Here's how the part is built. I have some questions about the finished solid (model axes, mm). A direction names the side the tool comes from. Round coordinates to 2 decimals unless told otherwise and drop trailing zeros. Write each loop counter-clockwise with the first axis right and the second up, starting at its lowest first coordinate (ties: lowest second). Pieces come first, ordered by that corner, then holes. Notation, with made-up numbers: (-38.75, 11.5) -> (-14.75, 11.5) arc R26 cw to (-14.75, 34.5) -> close; hole circle Ø10 at (49, -37.5). An arc over 180 degrees is marked (long way). Answer in a Markdown table with one row per item. Add a question column.
from build123d import *

# Parameters (mm, degrees)
SKETCH2_W           = 130
SKETCH2_H           = 70
BOSS_EXTRUDE1_DEPTH = 100
SKETCH3_W           = 104
SKETCH3_H           = 74
CUT_EXTRUDE1_DEPTH  = 67
SKETCH4_W           = 10
SKETCH4_H           = 10
CUT_EXTRUDE2_DEPTH  = 55
SKETCH5_W           = 104
SKETCH5_H           = 10
CUT_EXTRUDE3_DEPTH  = 67
SKETCH6_W           = 10
SKETCH6_H           = 74
CUT_EXTRUDE4_DEPTH  = 67
SKETCH9_R           = 1.75
CUT_EXTRUDE5_DEPTH  = 67
SKETCH10_R          = 4
CUT_EXTRUDE6_DEPTH  = 5
SKETCH12_R          = 4
CUT_EXTRUDE7_DEPTH  = 5
SKETCH13_R          = 4
CUT_EXTRUDE8_DEPTH  = 5
SKETCH14_R          = 4
CUT_EXTRUDE9_DEPTH  = 5
SKETCH15_W          = 3
SKETCH15_H          = 3
BOSS_EXTRUDE2_DEPTH = 5
SKETCH16_W          = 76
SKETCH16_H          = 3
BOSS_EXTRUDE3_DEPTH = 15
SKETCH17_W          = 3
SKETCH17_H          = 30
BOSS_EXTRUDE4_DEPTH = 15
SKETCH18_R          = 5.8
CUT_EXTRUDE10_DEPTH = 15
SKETCH19_R          = 3.4
CUT_EXTRUDE11_DEPTH = 15


with BuildPart() as part:
    # Sketch2 → Boss-Extrude1 (new body)
    with BuildSketch(Plane(origin=(0, 0, 0), x_dir=(1, 0, 0), z_dir=(0, 1, 0))):
        with Locations((65, 35)):
            Rectangle(SKETCH2_W, SKETCH2_H)
    extrude(amount=BOSS_EXTRUDE1_DEPTH)

    # Sketch3 → Cut-Extrude1 (cut)
    with BuildSketch(Plane(origin=(0, 0, -70), x_dir=(-1, 0, 0), z_dir=(0, 0, -1))):
        with Locations((-65, 50)):
            Rectangle(SKETCH3_W, SKETCH3_H)
    extrude(amount=-CUT_EXTRUDE1_DEPTH, mode=Mode.SUBTRACT)

    # Sketch4 → Cut-Extrude2 (cut)
    with BuildSketch(Plane.XY):
        with Locations((5, 95)):
            Rectangle(SKETCH4_W, SKETCH4_H)
        with Locations((125, 95)):
            Rectangle(SKETCH4_W, SKETCH4_H)
        with Locations((5, 5)):
            Rectangle(SKETCH4_W, SKETCH4_H)
        with Locations((125, 5)):
            Rectangle(SKETCH4_W, SKETCH4_H)
    extrude(amount=-CUT_EXTRUDE2_DEPTH, mode=Mode.SUBTRACT)

    # Sketch5 → Cut-Extrude3 (cut)
    with BuildSketch(Plane(origin=(0, 0, -70), x_dir=(-1, 0, 0), z_dir=(0, 0, -1))):
        with Locations((-65, 92)):
            Rectangle(SKETCH5_W, SKETCH5_H)
        with Locations((-65, 8)):
            Rectangle(SKETCH5_W, SKETCH5_H)
    extrude(amount=-CUT_EXTRUDE3_DEPTH, mode=Mode.SUBTRACT)

    # Sketch6 → Cut-Extrude4 (cut)
    with BuildSketch(Plane(origin=(0, 0, -70), x_dir=(-1, 0, 0), z_dir=(0, 0, -1))):
        with Locations((-122, 50)):
            Rectangle(SKETCH6_W, SKETCH6_H)
        with Locations((-8, 50)):
            Rectangle(SKETCH6_W, SKETCH6_H)
    extrude(amount=-CUT_EXTRUDE4_DEPTH, mode=Mode.SUBTRACT)

    # Sketch9 → Cut-Extrude5 (cut)
    with BuildSketch(Plane(origin=(0, 0, -70), x_dir=(-1, 0, 0), z_dir=(0, 0, -1))):
        with Locations((-124, 94)):
            Circle(SKETCH9_R)
        with Locations((-124, 6)):
            Circle(SKETCH9_R)
        with Locations((-6, 94)):
            Circle(SKETCH9_R)
        with Locations((-6, 6)):
            Circle(SKETCH9_R)
    extrude(amount=-CUT_EXTRUDE5_DEPTH, mode=Mode.SUBTRACT)

    # Sketch10 → Cut-Extrude6 (cut)
    with BuildSketch(Plane.XY.offset(-55)):
        with Locations((124, 94)):
            Circle(SKETCH10_R)
    extrude(amount=-CUT_EXTRUDE6_DEPTH, mode=Mode.SUBTRACT)

    # Sketch12 → Cut-Extrude7 (cut)
    with BuildSketch(Plane.XY.offset(-55)):
        with Locations((124, 6)):
            Circle(SKETCH12_R)
    extrude(amount=-CUT_EXTRUDE7_DEPTH, mode=Mode.SUBTRACT)

    # Sketch13 → Cut-Extrude8 (cut)
    with BuildSketch(Plane.XY.offset(-55)):
        with Locations((6, 6)):
            Circle(SKETCH13_R)
    extrude(amount=-CUT_EXTRUDE8_DEPTH, mode=Mode.SUBTRACT)

    # Sketch14 → Cut-Extrude9 (cut)
    with BuildSketch(Plane.XY.offset(-55)):
        with Locations((6, 94)):
            Circle(SKETCH14_R)
    extrude(amount=-CUT_EXTRUDE9_DEPTH, mode=Mode.SUBTRACT)

    # Sketch15 → Boss-Extrude2 (add)
    with BuildSketch(Plane(origin=(0, 0, -70), x_dir=(-1, 0, 0), z_dir=(0, 0, -1))):
        with Locations((-118.5, 88.5)):
            Rectangle(SKETCH15_W, SKETCH15_H)
        with Locations((-118.5, 11.5)):
            Rectangle(SKETCH15_W, SKETCH15_H)
        with Locations((-11.5, 11.5)):
            Rectangle(SKETCH15_W, SKETCH15_H)
        with Locations((-11.5, 88.5)):
            Rectangle(SKETCH15_W, SKETCH15_H)
    extrude(amount=BOSS_EXTRUDE2_DEPTH)

    # Sketch16 → Boss-Extrude3 (add)
    with BuildSketch(Plane(origin=(0, 3, 0), x_dir=(1, 0, 0), z_dir=(0, 1, 0))):
        with Locations((79, 68.5)):
            Rectangle(SKETCH16_W, SKETCH16_H)
    extrude(amount=BOSS_EXTRUDE3_DEPTH)

    # Sketch17 → Boss-Extrude4 (add)
    with BuildSketch(Plane(origin=(0, 0, -3), x_dir=(-1, 0, 0), z_dir=(0, 0, -1))):
        with Locations((-99.5, 33)):
            Rectangle(SKETCH17_W, SKETCH17_H)
        with Locations((-36.5, 33)):
            Rectangle(SKETCH17_W, SKETCH17_H)
    extrude(amount=BOSS_EXTRUDE4_DEPTH)

    # Sketch18 → Cut-Extrude10 (cut)
    with BuildSketch(Plane(origin=(0, 0, -3), x_dir=(-1, 0, 0), z_dir=(0, 0, -1))):
        with Locations((-20, 25)):
            Circle(SKETCH18_R)
    extrude(amount=-CUT_EXTRUDE10_DEPTH, mode=Mode.SUBTRACT)

    # Sketch19 → Cut-Extrude11 (cut)
    with BuildSketch(Plane(origin=(0, 100, 0), x_dir=(1, 0, 0), z_dir=(0, 1, 0))):
        with Locations((25, 45)):
            Circle(SKETCH19_R)
        with Locations((45, 45)):
            Circle(SKETCH19_R)
        with Locations((65, 45)):
            Circle(SKETCH19_R)
        with Locations((85, 45)):
            Circle(SKETCH19_R)
        with Locations((105, 45)):
            Circle(SKETCH19_R)
    extrude(amount=-CUT_EXTRUDE11_DEPTH, mode=Mode.SUBTRACT)


solid = part.part
Item 1: I need wall thicknesses on line 1 along X through (y, z) = (99.3, -45); line 2 along X through (y, z) = (38, -17.5); line 3 along X through (y, z) = (54, -17). Which ranges of each line are inside material? Lowest first, please. Write a range as from..to.
Item 2: If we section it at C-C on x = 65: Please give me the cut outline in (y, z).
Item 3: If we section it at A-A on z = -15: Give the number of separate pieces and of enclosed holes in the cut face, then the cut area to 3 significant figures.
Item 4: For P1, Ø8, axis at x = 125, y = 95, coming from the +Z side; P2, Ø5, axis at x = 3, z = -15.5, coming from the -Y side; P3, Ø1, axis at x = 68, y = 12, coming from the -Z side, each with a flat end and sliding along its axis, tell me the tip position at first contact or that it passes through.
Item 5: If we mould it in two halves opening along X, with no side actions, what happens to faces 6 (the flat face through (5, 90, -27)), 7 (the flat face through (41, 10, -68)), 8 (the flat face through (120, 88, -72))? For each: pulls with the +X half, pulls with the -X half, needs draft (parallel to the pull), parting line crosses it, or undercut.
Item 6: If we section it at B-B on y = 25: Please give me the cut outline in (x, z).
Item 7: On a 3-axis mill with a long thin cutter (end or side, diameter ignored), from which of +Z, -Z, +X, -X, +Y, -Y can I reach the whole of each face in a straight line? I mean faces 1 (the flat face through (10, 11, -72)), 2 (the flat face through (9, 91, -55)), 3 (the flat face through (37, 33, -18)), 4 (the flat face through (66, 3, -37)), 5 (the flat face through (120, 5, -27)). Say none if no direction works.
Item 8: If we section it at D-D on y = 65.5: Please give me the cut outline in (x, z), then the cut area to 3 significant figures.
Results list:
| question | item | result |
|---|---|---|
| 1 | line 1 | 10..21.6, 28.4..41.6, 48.4..61.6, 68.4..81.6, 88.4..101.6, 108.4..120 |
| 1 | line 2 | 0..3, 35..38, 98..101, 127..130 |
| 1 | line 3 | 0..3, 127..130 |
| 2 | outline | (0, -70) -> (18, -70) -> (18, -67) -> (3, -67) -> (3, -3) -> (97, -3) -> (97, -41.6) -> (100, -41.6) -> (100, 0) -> (0, 0) -> close; (97, -70) -> (100, -70) -> (100, -48.4) -> (97, -48.4) -> close |
| 3 | separate pieces | 3 |
| 3 | enclosed holes | 1 |
| 3 | area | 1,520 mm² |
| 4 | P1 | z = -55 |
| 4 | P2 | y = 10 |
| 4 | P3 | z = -70 |
| 5 | face 6 | needs draft |
| 5 | face 7 | undercut |
| 5 | face 8 | pulls with the +X half |
| 6 | outline | (0, -70) -> (3, -70) -> (3, -3) -> (14.2, -3) -> (14.2, 0) -> (0, 0) -> close; (25.8, -3) -> (35, -3) -> (35, -18) -> (38, -18) -> (38, -3) -> (98, -3) -> (98, -18) -> (101, -18) -> (101, -3) -> (127, -3) -> (127, -70) -> (130, -70) -> (130, 0) -> (25.8, 0) -> close |
| 7 | face 1 | -Z, -X, +Y, -Y |
| 7 | face 2 | +Z, -X, +Y |
| 7 | face 3 | -Z |
| 7 | face 4 | none |
| 7 | face 5 | +Z, +X, -Y |
| 8 | outline | (0, -70) -> (3, -70) -> (3, -3) -> (127, -3) -> (127, -70) -> (130, -70) -> (130, 0) -> (0, 0) -> close |
| 8 | area | 792 mm² |
